Geometry: see drawing. Coordinates: mm, zero at the bounding-box minimum. Give positions to 0.01 mm unless a question says otherwise; leave off trailing zeros. Write each loop counter-clockwise with the first axis right and the second up, starting at its lowest first coordinate (ties: lowest second). Pieces come first, ordered by that corner, then holes. Notation, with made-up numbers: M 39.5,40 L 97.5,40 A25 ccw 97.5,67 Z; hole C 3.25,54 d5. An arc over 180 degrees is marked long. Use a Markdown table: item, result. Add a question column.
1) Pin query (flat end, axial travel): pin 1 (6 mm diameter, centred on x = 8, y = 41, fed in from -Z); pin 2 (14.5 mm diameter, centred on x = 27, y = 15, fed in from -Z) (3 decimals). Return the tip coordinate at first contact, or that it passes through.
2) Section B-B on y = 41. Return the cut outline in (x, z), then the cut area to 3 significant figures.
3) Line query: line 1 (Y direction, x = 8, z = 0.65); line 2 (X direction, y = 40, z = 1.05); line 3 (Y direction, x = 27, z = 1.25). Output: solid intervals per line, ascending.
4) Section A-A on x = 27. Return the cut outline in (y, z), then the cut area to 3 significant figures.
5) Section D-D on z = 1.3. State how many separate pieces and enclosed holes the cut face has, then the cut area to 3 significant figures.
6) Section C-C on y = 15. Return the cut outline in (x, z).
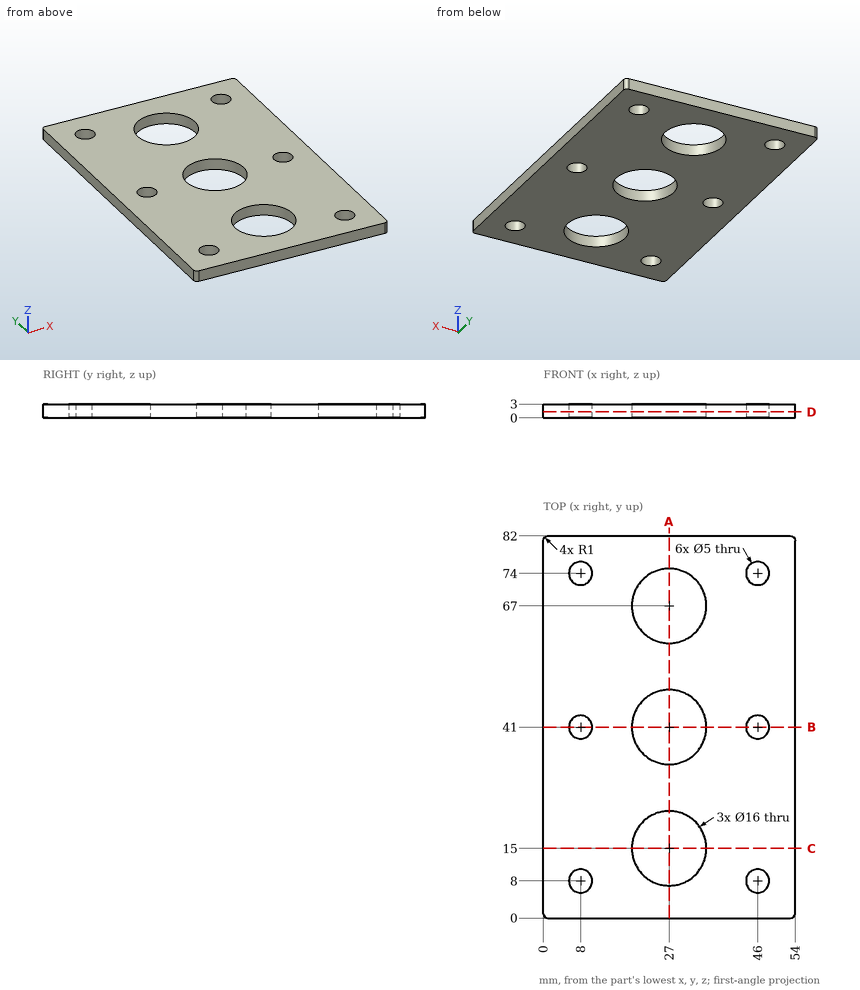
Found:
| question | item | result |
|---|---|---|
| 1 | pin 1 | z = 0 |
| 1 | pin 2 | through |
| 2 | outline | M 0,0 L 5.5,0 L 5.5,3 L 0,3 Z; M 10.5,0 L 19,0 L 19,3 L 10.5,3 Z; M 35,0 L 43.5,0 L 43.5,3 L 35,3 Z; M 48.5,0 L 54,0 L 54,3 L 48.5,3 Z |
| 2 | area | 84.0 mm² |
| 3 | line 1 | 0 to 5.5, 10.5 to 38.5, 43.5 to 71.5, 76.5 to 82 |
| 3 | line 2 | 0 to 5.71, 10.29 to 19.06, 34.94 to 43.71, 48.29 to 54 |
| 3 | line 3 | 0 to 7, 23 to 33, 49 to 59, 75 to 82 |
| 4 | outline | M 0,0 L 7,0 L 7,3 L 0,3 Z; M 23,0 L 33,0 L 33,3 L 23,3 Z; M 49,0 L 59,0 L 59,3 L 49,3 Z; M 75,0 L 82,0 L 82,3 L 75,3 Z |
| 4 | area | 102 mm² |
| 5 | separate pieces | 1 |
| 5 | enclosed holes | 9 |
| 5 | area | 3,710 mm² |
| 6 | outline | M 0,0 L 19,0 L 19,3 L 0,3 Z; M 35,0 L 54,0 L 54,3 L 35,3 Z |
